Verification items for the finished model (mm, model axes). A direction names the side the tool comes from. Give positions to 0.01 mm unless a question says otherwise; leave off trailing zeros. Order: outer loops, then holes, each group sorted by start corner. A loop starts at its lowest first (then second) coordinate and runs counter-clockwise, first axis right, second up.
from build123d import *

# Parameters (mm, degrees)
F0_W     = 70
F0_H     = 10
F1_DEPTH = 5
F2_R     = 4.99999


# Not quite as in the source:
# - a fillet or chamfer is up to 0.001 mm smaller than in the source, because OpenCascade refuses the exact size


with BuildPart() as f1:
    # F0 (on Top) → F1 (new body)
    with BuildSketch(Plane.XY):
        Polygon((300, 149.2274475843), (-300, 149.2274475843), (-300, -150.7725524157), (300, -150.7725524157), (300, -75.7725524157), (250, -75.7725524157), (201.9998562336, -95.7725524157), (131.9998562336, -95.7725524157), (131.9998562336, -85.7725524157), (201.9998562336, -85.7725524157), (250, -65.7725524157), (300, -65.7725524157), (300, -30.7725524157), (250, -30.7725524157), (250, 29.2274475843), (300, 29.2274475843), (300, 64.2274475843), (250, 64.2274475843), (201.9998562336, 84.2274475843), (131.9998562336, 84.2274475843), (131.9998562336, 94.2274475843), (201.9998562336, 94.2274475843), (250, 74.2274475843), (300, 74.2274475843), align=None)
        with Locations((-233.0001437664, -90.7725524157)):
            Rectangle(F0_W, F0_H, mode=Mode.SUBTRACT)
        with Locations((-133.0001437664, -90.7725524157)):
            Rectangle(F0_W, F0_H, mode=Mode.SUBTRACT)
        with Locations((-33.0001437664, -90.7725524157)):
            Rectangle(F0_W, F0_H, mode=Mode.SUBTRACT)
        with Locations((66.9998562336, -90.7725524157)):
            Rectangle(F0_W, F0_H, mode=Mode.SUBTRACT)
        with Locations((-233.0001437664, 89.2274475843)):
            Rectangle(F0_W, F0_H, mode=Mode.SUBTRACT)
        with Locations((-133.0001437664, 89.2274475843)):
            Rectangle(F0_W, F0_H, mode=Mode.SUBTRACT)
        with Locations((-33.0001437664, 89.2274475843)):
            Rectangle(F0_W, F0_H, mode=Mode.SUBTRACT)
        with Locations((66.9998562336, 89.2274475843)):
            Rectangle(F0_W, F0_H, mode=Mode.SUBTRACT)
    extrude(amount=F1_DEPTH)

    # F2 (radius 5 in the source; OpenCascade refuses exactly that, so slightly less here)
    f2_edges = [f1.edges().sort_by_distance(p)[0] for p in [
        (131.999856, -95.772552, 2.5),
        (31.999856, -95.772552, 2.5),
        (-68.000144, -95.772552, 2.5),
        (201.999856, -95.772552, 2.5),
        (250, -75.772552, 2.5),
        (-168.000144, -95.772552, 2.5),
        (-268.000144, -95.772552, 2.5),
        (300, -75.772552, 2.5),
        (300, -65.772552, 2.5),
        (300, -30.772552, 2.5),
        (250, -30.772552, 2.5),
        (250, -65.772552, 2.5),
        (201.999856, -85.772552, 2.5),
        (131.999856, -85.772552, 2.5),
        (101.999856, -85.772552, 2.5),
        (1.999856, -85.772552, 2.5),
        (-98.000144, -85.772552, 2.5),
        (-198.000144, -85.772552, 2.5),
        (31.999856, -85.772552, 2.5),
        (-68.000144, -85.772552, 2.5),
        (-168.000144, -85.772552, 2.5),
        (-268.000144, -85.772552, 2.5),
        (101.999856, -95.772552, 2.5),
        (1.999856, -95.772552, 2.5),
        (-98.000144, -95.772552, 2.5),
        (-198.000144, -95.772552, 2.5),
    ]]
    fillet(f2_edges, radius=F2_R)


solid = f1.part
(1) Release check for a two-part mould opening along Y. For faces 1 (the flat face through (226.32, -85.64, 2.46)), 2 (the flat face through (-4, 1, 5)), 3 (the flat face through (226.336, 74.087, 2.465)) record: pulls with the +Y half, pulls with the -Y half, needs draft (parallel to the pull), parting line crosses it, or undercut.
Solved:
face 1: undercut
face 2: needs draft
face 3: undercut
(2) Section check B-B, the plane z = 2.85. Give the number of separate pieces and of enclosed holes in the cut face, then the cut area to 3 significant figures.
Solved:
separate pieces: 1
enclosed holes: 8
area: 168,000 mm2
(3) Section check A-A, the plane x = 164. Enter the section's corners in (y, z), then the cut area to 3 significant figures.
Solved:
outline: (-150.77, 0) - (-95.77, 0) - (-95.77, 5) - (-150.77, 5) - close; (-85.77, 0) - (84.23, 0) - (84.23, 5) - (-85.77, 5) - close; (94.23, 0) - (149.23, 0) - (149.23, 5) - (94.23, 5) - close
area: 1,400 mm2
(4) Scan lines: line 1 (Y direction, x = 178.5, z = 3.05); line 2 (Y direction, x = 136, z = 1.3); line 3 (Y direction, x = 263, z = 0.8). Record each from-to range of solid material in increasing order.
Solved:
line 1: y = -150.77 to -95.77, -85.77 to 84.23, 94.23 to 149.23
line 2: y = -150.77 to -95.67, -85.87 to 84.23, 94.23 to 149.23
line 3: y = -150.77 to -75.77, -65.77 to -30.77, 29.23 to 64.23, 74.23 to 149.23
(5) Set-up check for faces 4 (the flat face through (225.677, -75.907, 2.465)), 5 (the flat face through (-4, 1, 0)): record each of +Z, -Z, +X, -X, +Y, -Y from which the full face is reachable in a straight line by a thin tool's end or side.
Solved:
face 4: +Z, -Z
face 5: -Z, +X, -X, +Y, -Y
(6) Section check C-C, the plane y = 3.5. Enter the section's corners in (x, z).
Solved:
outline: (-300, 0) - (250, 0) - (250, 5) - (-300, 5) - close
(7) Go/stop test with a flat-tipped pin: pin 1 (1 mm diameter, centred on x = 231, y = -83, fed in from -Z). Record where the tip stops, or that it passes through.
Solved:
pin 1: passes through
